The figure shows three views and two pictorial views of one solid part (mm, origin at its lowest corner). Answer the questions. A direction names the side the tool comes from. Give positions to 0.01 mm unless a question says otherwise; leave off trailing zeros. Loops run counter-clockwise (first coordinate to the right, second up) from the corner with the lowest first, then second, coordinate; pieces in that order, holes last. Notation, with made-up numbers: M 32.25,72.25 L 68.25,72.25 A35 ccw 68.25,104.25 Z; hole C 6.5,-9.5 d9. An arc over 180 degrees is marked long. Write item = value, one per line. Start each with the question number.
1. Section B-B on z = 4.5 is taken. Determine the outline of the cut face in (x, y), plus the area to 3 significant figures.
2. Consider L1, parallel to X at y = 26, z = 4; L2, parallel to Y at x = 60, z = 20; L3, parallel to X at y = 40.5, z = 38. Determine where each line is inside the solid, lowest interval first. Write a range as [from, to].
3. The mould has two halves that part along X. Classify the marked faces 1, 2 and 3: released by +X, released by -X, zero draft, split by the parting line, or undercut.
4. Section C-C on y = 12 is taken. Determine the outline of the cut face in (x, z), plus the area to 3 significant figures.
5. Section A-A on y = 42.5 is taken. Determine the outline of the cut face in (x, z).
6. Flat-ended cylindrical pins translate along their axes: pin 1 Ø15 at (y, z) = (41.5, 39.5) entering from +X; pin 2 Ø10 at (x, z) = (46, 28) entering from +Y. Find the tip coordinate at first contact, or state that the pin passes through.
7. Section D-D on x = 38 is taken. Determine the outline of the cut face in (y, z), plus the area to 3 significant figures.
8. For the marked faces 4 and 5, determine the directions among +Z, -Z, +X, -X, +Y, -Y from which every point of the face is accessible in a straight line to the end or side of a thin tool.
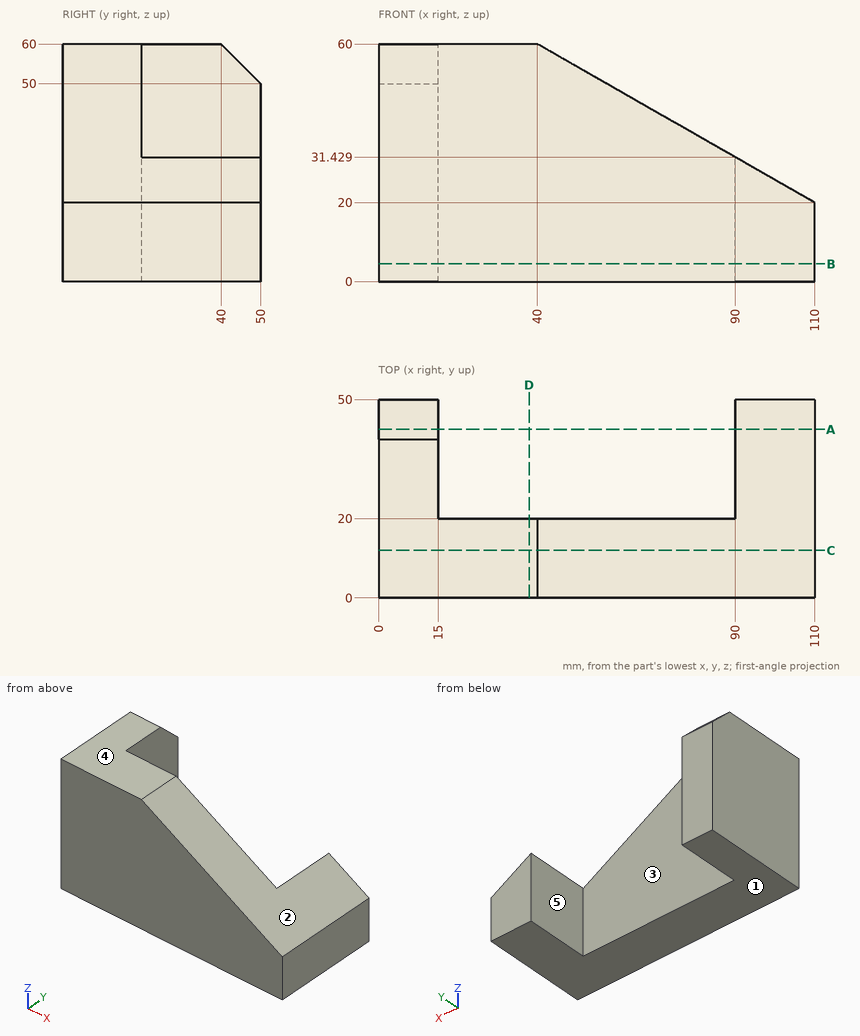
Verdict:
q1.outline = M 0,0 L 110,0 L 110,50 L 90,50 L 90,20 L 15,20 L 15,50 L 0,50 Z
q1.area = 3,250 mm2
q2.L1 = [0, 15], [90, 110]
q2.L2 = [0, 20]
q2.L3 = [0, 15]
q3.face_1 = zero draft
q3.face_2 = released by +X
q3.face_3 = undercut
q4.outline = M 0,0 L 110,0 L 110,20 L 40,60 L 0,60 Z
q4.area = 5,200 mm2
q5.outline = M 0,0 L 15,0 L 15,57.5 L 0,57.5 Z; M 90,0 L 110,0 L 110,20 L 90,31.43 Z
q6.pin_1 = 15
q6.pin_2 = 20
q7.outline = M 0,0 L 20,0 L 20,60 L 0,60 Z
q7.area = 1,200 mm2
q8.face_4 = +Z, +X, -X, +Y, -Y
q8.face_5 = +Z, -Z, +Y
